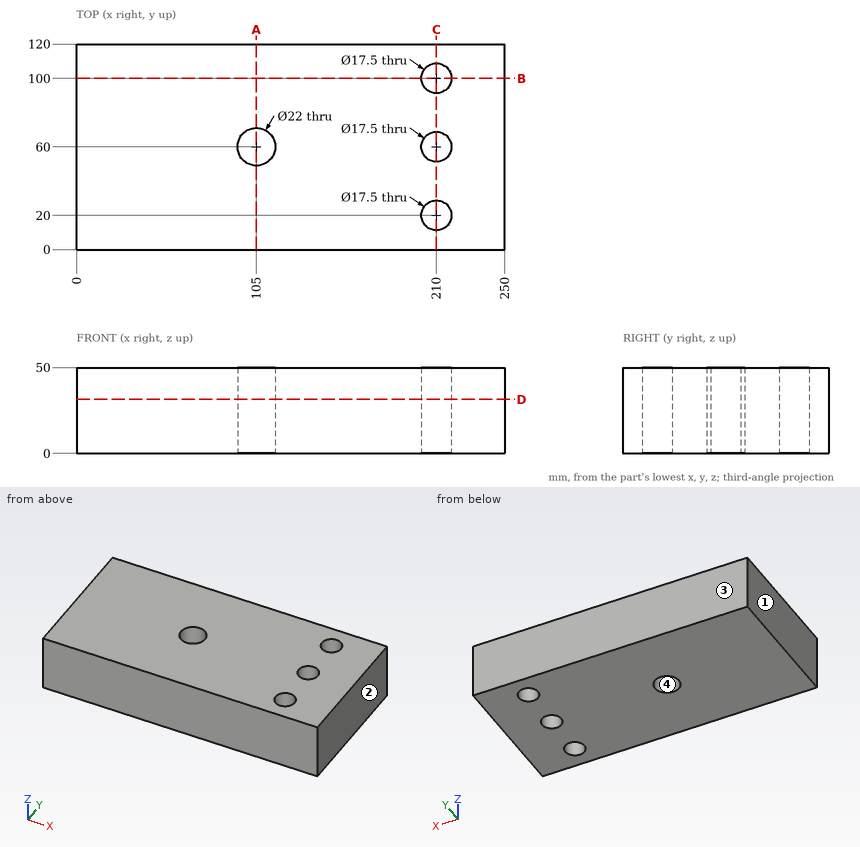
Design review of the part shown in the three views and the two pictorial views. Dimensions are in mm from the part's minimum x, y and z. Round coordinates to 2 decimals unless told otherwise and drop trailing zeros. Loops run counter-clockwise (first coordinate to the right, second up) from the corner with the lowest first, then second, coordinate; pieces in that order, holes last.
Q1. Mouldability with a two-part tool opening along X and no side actions: class the marked faces 1, 2, 3 and 4 as +X half, -X half, draft (parallel to the pull), parting line (faces both ways), or undercut.
Result sheet:
face 1: -X half
face 2: +X half
face 3: draft
face 4: undercut
Q2. Insertion check: pin 1 Ø10.5 at (x, y) = (210, 60) entering from -Z. The pin has a flat end and moves straight along its axis. Give the tip position at first contact, or say it passes through.
Result sheet:
pin 1: passes through
Q3. Add section B-B on y = 100. Write out the cut boundary in (x, z), plus the area to 3 significant figures.
Result sheet:
outline: (0, 0) - (201.25, 0) - (201.25, 50) - (0, 50) - close; (218.75, 0) - (250, 0) - (250, 50) - (218.75, 50) - close
area: 11,600 mm2
Q4. Add section D-D on z = 31.5. Write out the cut boundary in (x, y), plus the area to 3 significant figures.
Result sheet:
outline: (0, 0) - (250, 0) - (250, 120) - (0, 120) - close; hole circle Ø22 at (105, 60); hole circle Ø17.5 at (210, 20); hole circle Ø17.5 at (210, 60); hole circle Ø17.5 at (210, 100)
area: 28,900 mm2
Q5. To check wall thickness, follow line 1 along Y through (x, z) = (210, 19); line 2 along X through (y, z) = (59.5, 45); line 3 along Y through (x, z) = (206.5, 31). State the ranges of each line that lie inside material, in increasing order.
Result sheet:
line 1: y = 0 to 11.25, 28.75 to 51.25, 68.75 to 91.25, 108.75 to 120
line 2: x = 0 to 94.01, 115.99 to 201.26, 218.74 to 250
line 3: y = 0 to 11.98, 28.02 to 51.98, 68.02 to 91.98, 108.02 to 120
Q6. Add section C-C on x = 210. Write out the cut boundary in (y, z).
Result sheet:
outline: (0, 0) - (11.25, 0) - (11.25, 50) - (0, 50) - close; (28.75, 0) - (51.25, 0) - (51.25, 50) - (28.75, 50) - close; (68.75, 0) - (91.25, 0) - (91.25, 50) - (68.75, 50) - close; (108.75, 0) - (120, 0) - (120, 50) - (108.75, 50) - close
Q7. Add section A-A on x = 105. Write out the cut boundary in (y, z).
Result sheet:
outline: (0, 0) - (49, 0) - (49, 50) - (0, 50) - close; (71, 0) - (120, 0) - (120, 50) - (71, 50) - close
